Read the model definition and answer for the solid it produces. Units are mm, in the model's axes. Face numbers are marked on the shaded views. Give positions to 0.01 mm unless a question says otherwise; leave off trailing zeros. Loops run counter-clockwise (first coordinate to the right, second up) from the corner with the lowest first, then second, coordinate; pieces in that order, holes last. Notation, with made-up numbers: (74.5, -0.5) -> (132.5, -0.5) arc R6 ccw to (132.5, 7.5) -> close; hole circle Ø6 at (76, -5.5). An arc over 180 degrees is marked (long way). Write each question's results on one line, items separated by ' | '. Start each with the question number.
Item 1: Section C-C on z = 9.25 is taken. Write down the section's boundary in (x, y), and give its area (3 significant figures).
Item 2: This flat-tipped pin is pushed along its axis until it touches: P1, Ø3, axis at x = -4.25, z = 11.25, coming from the +Y side. Where does it stop, or does it pass through?
Item 3: Section A-A on y = -2.75 is taken. Write down the section's boundary in (x, z), and give its area (3 significant figures).
Item 4: Section D-D on z = 11.25 is taken. Write down the section's boundary in (x, y), and give its area (3 significant figures).
Item 5: Determine the mould class of the marked faces 1, 2 and 3 for opening direction Z: +Z half, -Z half, draft (parallel to the pull), parting line (faces both ways), or undercut.
Item 6: Section B-B on x = -5.25 is taken. Write down the section's boundary in (y, z), and give its area (3 significant figures).
Item 7: Find the intervals of material crossed by line 1 (Z direction, x = -4.25, y = -2.3); line 2 (Z direction, x = 3, y = -0.5); line 3 (X direction, y = -2.6, z = 11.25), in increasing order.
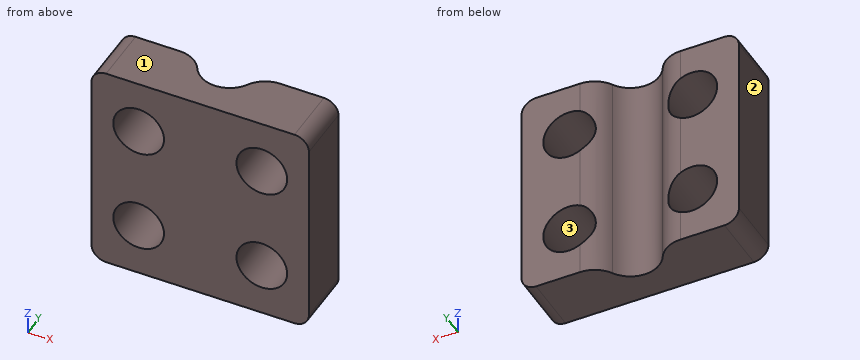
```python
from build123d import *

# Parameters (mm, degrees)
F0_W         = 15
F0_H         = 8
F2_DEPTH     = 15
F1_R         = 2
F3_DEPTH     = 20
F4_R         = 1.75
F5_DEPTH     = 15
F6_DEPTH     = 25
F8_R         = 1.75
F9_DEPTH     = 25
F10_R        = 1.75
F11_DEPTH    = 25
F7_W         = 19.053414464
F7_H         = 8.769848384
F12_DEPTH    = 25
F13_T1_DEPTH = 22.3205080757
F14_R        = 1


# Not quite as in the source:
# - a fillet or chamfer that OpenCascade refuses, or shapes differently, is made with other operations: its cross-section is extruded or revolved along the edge and cut away or added


with BuildPart() as f2:
    # F0 (on Top) → F2 (new body)
    with BuildSketch(Plane.XY):
        Rectangle(F0_W, F0_H)
    extrude(amount=F2_DEPTH)

    # F1 (on Top) → F3 (cut)
    with BuildSketch(Plane.XY):
        Circle(F1_R)
    extrude(amount=F3_DEPTH, mode=Mode.SUBTRACT)

    # F4 (on Front) → F5 (cut)
    with BuildSketch(Plane.XZ):
        with Locations((-4.25, 11.25)):
            Circle(F4_R)
    extrude(amount=F5_DEPTH, mode=Mode.SUBTRACT)

    # F4 (on Front) → F6 (cut)
    with BuildSketch(Plane.XZ):
        with Locations((-4.25, 11.25)):
            Circle(F4_R)
    extrude(amount=-F6_DEPTH, mode=Mode.SUBTRACT)

    # F8 (on face) → F9 (cut)
    with BuildSketch(Plane.XZ.offset(4)):
        with Locations((-4.25, 3.75)):
            Circle(F8_R)
    extrude(amount=-F9_DEPTH, mode=Mode.SUBTRACT)

    # F10 (on face) → F11 (cut)
    with BuildSketch(Plane.XZ.offset(4)):
        with Locations((4.25, 11.25)):
            Circle(F10_R)
        with Locations((4.25, 3.75)):
            Circle(F10_R)
    extrude(amount=-F11_DEPTH, mode=Mode.SUBTRACT)

    # F7 (on Top) → F12 (cut)
    with BuildSketch(Plane.XY):
        with Locations((0, 4.384924192)):
            Rectangle(F7_W, F7_H)
    extrude(amount=F12_DEPTH, mode=Mode.SUBTRACT)

    # F13: fillet of radius 2 on 2 edges, made by hand

    # F13_s2 → F13_t1 (cut)
    with BuildSketch(Plane.XY.offset(-3.6602540378)):
        with BuildLine():
            ThreePointArc((1.7320508076, -1), (2.4641016151, -0.2679491924), (3.4641016151, 0))
            Line((3.4641016151, 0), (2, 0))
            ThreePointArc((2, 0), (1.9318516526, -0.5176380902), (1.7320508076, -1))
        make_face()
        with BuildLine():
            ThreePointArc((-3.4641016151, 0), (-2.4641016151, -0.2679491924), (-1.7320508076, -1))
            ThreePointArc((-1.7320508076, -1), (-1.9318516526, -0.5176380902), (-2, 0))
            Line((-2, 0), (-3.4641016151, 0))
        make_face()
    extrude(amount=F13_T1_DEPTH, mode=Mode.SUBTRACT)

    # F14
    f14_edges = [f2.edges().sort_by_distance(p)[0] for p in [
        (-7.5, -2, 15),
        (-7.5, -2, 0),
        (7.5, -2, 15),
        (7.5, -2, 0),
    ]]
    fillet(f14_edges, radius=F14_R)


solid = f2.part
```
Findings:
1) outline: (-7.5, -4) -> (7.5, -4) -> (7.5, 0) -> (3.46, 0) arc R2 ccw to (1.73, -1) arc R2 cw to (-1.73, -1) arc R2 ccw to (-3.46, 0) -> (-7.5, 0) -> close | area: 53.1 mm2
2) P1: through
3) outline: (-7.5, 1) arc R1 ccw to (-6.5, 0) -> (6.5, 0) arc R1 ccw to (7.5, 1) -> (7.5, 14) arc R1 ccw to (6.5, 15) -> (-6.5, 15) arc R1 ccw to (-7.5, 14) -> close; hole circle Ø3.5 at (-4.25, 3.75); hole circle Ø3.5 at (-4.25, 11.25); hole circle Ø3.5 at (4.25, 3.75); hole circle Ø3.5 at (4.25, 11.25) | area: 186 mm2
4) outline: (-7.5, -4) -> (-6, -4) -> (-6, 0) -> (-7.5, 0) -> close; (-2.5, -4) -> (2.5, -4) -> (2.5, -0.25) arc R2 ccw to (1.73, -1) arc R2 cw to (-1.73, -1) arc R2 ccw to (-2.5, -0.25) -> close; (6, -4) -> (7.5, -4) -> (7.5, 0) -> (6, 0) -> close | area: 25.2 mm2
5) face 1: +Z half | face 2: draft | face 3: undercut
6) outline: (-4, 0) -> (0, 0) -> (0, 2.31) -> (-4, 2.31) -> close; (-4, 5.19) -> (0, 5.19) -> (0, 9.81) -> (-4, 9.81) -> close; (-4, 12.69) -> (0, 12.69) -> (0, 15) -> (-4, 15) -> close | area: 37.0 mm2
7) line 1: 0 to 2, 5.5 to 9.5, 13 to 15 | line 2: 0 to 2.53, 4.97 to 10.03, 12.47 to 15 | line 3: -7.5 to -6, -2.5 to 2.5, 6 to 7.5
